Build history of the part. All positions in model axes, mm. Face numbers are marked on the shaded views. A direction names the side the tool comes from. Give positions to 0.01 mm unless a question says otherwise; leave off trailing zeros. Loops run counter-clockwise (first coordinate to the right, second up) from the corner with the lowest first, then second, coordinate; pieces in that order, holes last.
1) Band-saw the part on B-B on x = 11. List the corners of the cut face in (y, z), then the cut area to 3 significant figures.
2) Band-saw the part on D-D on y = -3.5. List the corners of the cut face in (x, z).
3) 3-axis set-ups, long thin cutter, end or side, ignore diameter. For the marked faces 5 and 6: which of +Z, -Z, +X, -X, +Y, -Y reach the whole face in a straight line?
4) Flat gauge pins, fed straight in: P1, Ø2, axis at x = 22.5, y = -2.5, coming from the -Z side; P2, Ø5, axis at y = 1, z = 0.5, coming from the -X side; P3, Ø3, axis at x = 0, z = 0, coming from the -Y side. Where does each tip first touch, or does it go through?
5) Wall check: line 1 (Z direction, x = 14.5, y = 3.25); line 2 (Z direction, x = 0, y = -7); line 3 (X direction, y = -6.9, z = 0). Give the ranges that are in metal, low to high.
6) Two-plate mould, pull along Y, no slides. Class the marked faces 1, 2, 3 and 4: +Y half, -Y half, draft (parallel to the pull), parting line (faces both ways), or undercut.
7) Band-saw the part on A-A on z = 0. List the corners of the cut face in (x, y), then the cut area to 3 significant figures.
8) Band-saw the part on C-C on x = 0. List the corners of the cut face in (y, z).
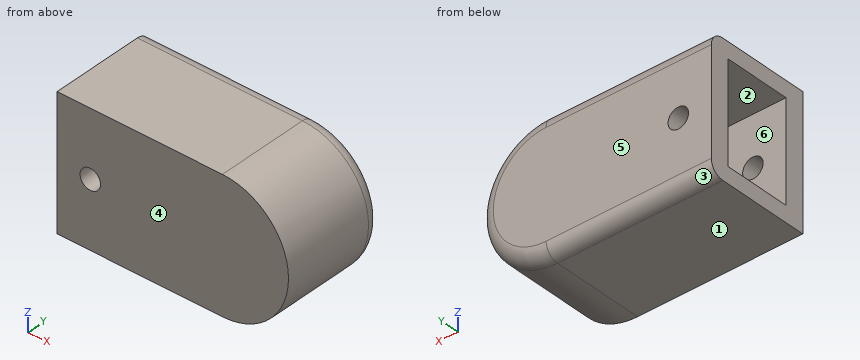
Autodesk Inventor part; units mm, degrees
ref_plane "YZ Plane" through (0, 0, 0) normal (1, 0, 0) x (0, 1, 0)
ref_plane "XZ Plane" through (0, 0, 0) normal (0, 1, 0) x (-1, 0, 0)
ref_plane "XY Plane" through (0, 0, 0) normal (0, 0, 1) x (1, 0, 0)
sketch "Sketch1" plane through (0, 0, 0) normal (0, 1, 0) x (-1, 0, 0)
  line L0 (5, -10) -> (-20, -10)
  line L1 (-20, -10) -> (-20, 10)
  line L2 (-20, 10) -> (5, 10)
  line L3 (5, 10) -> (5, -10)
  line L4 (5, -10) -> (-20, 10) construction
  line L5 (-20, -10) -> (5, 10) construction
  circle A0 centre (-20, 0) radius 10
  point P0 (0, 0)
  point P1 (-7.5, 0)
  point P2 (-20, 10)
  dimension "d0" = 20
  dimension "d1" = 20
  dimension "d2" = 5
extrude "Extrusion1" add sketch "Sketch1" along normal mid plane 16
sketch "Sketch2" plane through (0, 8, 0) normal (0, 1, 0) x (1, 0, 0)
  point P0 (0, 0)
  point P1 (0, 0)
hole "Hole1" at (0, 8, 0) direction (0, -1, 0) diameter 3.1 end through all
sketch "Sketch3" plane through (-5, -8, 10) normal (-1, 0, 0) x (0, 0, 1)
  line L0 (-17.56, 2.94) -> (-2.44, 2.94)
  line L1 (-2.44, 2.94) -> (-2.44, 13.06)
  line L2 (-2.44, 13.06) -> (-17.56, 13.06)
  line L3 (-17.56, 13.06) -> (-17.56, 2.94)
  line L4 (-17.56, 2.94) -> (-2.44, 13.06) construction
  line L5 (-2.44, 2.94) -> (-17.56, 13.06) construction
  point P0 (-10, 8)
  dimension "d12" = 15.12
  dimension "d13" = 10.12
extrude "Extrusion2" cut sketch "Sketch3" against normal blind 20.5
fillet "Fillet1" radius 2 3 edges at (30, 8, 0) (7.5, 8, -10) (7.5, 8, 10)
properties part number "T-Frame Right Cover" material "ABS Plastic"
Findings below:
1. outline: (-8, -10) - (6, -10) arc R2 ccw to (8, -8) - (8, 8) arc R2 ccw to (6, 10) - (-8, 10) - close; hole (-5.06, -7.56) - (5.06, -7.56) - (5.06, 7.56) - (-5.06, 7.56) - close
1. area: 165 mm2
2. outline: (-5, -10) - (20, -10) arc R10 ccw to (20, 10) - (-5, 10) - (-5, 7.56) - (15.5, 7.56) - (15.5, -7.56) - (-5, -7.56) - close
3. face 5: +Z, -Z, +X, -X, +Y
3. face 6: -X
4. P1: stops at z = -9.89
4. P2: stops at x = 15.5
4. P3: passes through
5. line 1: z = -10 to -7.56, 7.56 to 10
5. line 2: z = -10 to -1.55, 1.55 to 10
5. line 3: x = -5 to -1.55, 1.55 to 30
6. face 1: draft
6. face 2: undercut
6. face 3: +Y half
6. face 4: -Y half
7. outline: (-5, -8) - (-1.55, -8) - (-1.55, -5.06) - (-5, -5.06) - close; (-5, 5.06) - (-1.55, 5.06) - (-1.55, 8) - (-5, 8) - close; (1.55, -8) - (30, -8) - (30, 6) arc R2 ccw to (28, 8) - (1.55, 8) - (1.55, 5.06) - (15.5, 5.06) - (15.5, -5.06) - (1.55, -5.06) - close
7. area: 333 mm2
8. outline: (-8, -10) - (6, -10) arc R2 ccw to (8, -8) - (8, -1.55) - (5.06, -1.55) - (5.06, -7.56) - (-5.06, -7.56) - (-5.06, -1.55) - (-8, -1.55) - close; (-8, 1.55) - (-5.06, 1.55) - (-5.06, 7.56) - (5.06, 7.56) - (5.06, 1.55) - (8, 1.55) - (8, 8) arc R2 ccw to (6, 10) - (-8, 10) - close
